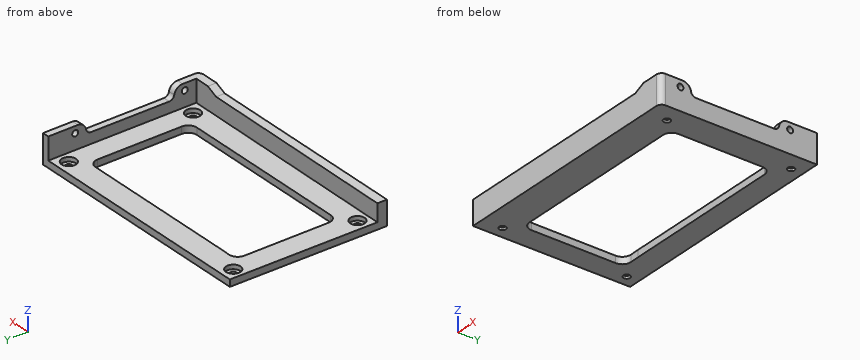
from build123d import *

# Parameters (mm, degrees)
F1_DEPTH  = 17
F3_DEPTH  = 13
F5_R      = 1.75
F6_DEPTH  = 7
F8_DEPTH  = 25
F9_R      = 3
F10_R     = 5
F11_R     = 2
F12_DEPTH = 25
F13_R     = 4.25
F14_DEPTH = 2.5
F16_DEPTH = 25
F17_R     = 5
F18_R     = 3


# Not quite as in the source:
# - ends of sketch curves that miss each other by under 0.0002 mm in the source are joined
# - a feature names something its author has since deleted; it is built from what else it names


with BuildPart() as f1:
    # F0 (on Top) → F1 (new body)
    with BuildSketch(Plane.XY):
        Polygon((67.6393576576, 43.5), (-74.3606423424, 43.5), (-74.7787490059, -48.5), (67.6393576576, -48.5), align=None)
    extrude(amount=F1_DEPTH)

    # F2 (on face) → F3 (cut)
    with BuildSketch(Plane.XY.offset(17)):
        Polygon((63.6393576576, 43.5), (-74.3606423424, 43.5), (-74.7531674957, -42.8710561201), (63.6393576576, -43.5), align=None)
    extrude(amount=-F3_DEPTH, mode=Mode.SUBTRACT)

    # F5 (on face) → F6 (cut)
    with BuildSketch(Plane.YZ.offset(67.6393576576)):
        with Locations((27.6843051805, 13.0568410139)):
            Circle(F5_R)
        with Locations((-36.7146101537, 13.0568410233)):
            Circle(F5_R)
        with BuildLine():
            ThreePointArc((27.6607478596, 17.0567716449), (27.6840839728, 17.0568410078), (27.7074200936, 17.0567742259))
            Line((27.7074200936, 17.0567742259), (47.12958325, 17.057848309))
            Line((47.12958325, 17.057848309), (47.1295543691, 17.7527777587))
            Line((47.1295543691, 17.7527777587), (48.6345604738, 26.1808149253))
            Line((48.6345604738, 26.1808149253), (32.3804893276, 26.9834864621))
            Line((32.3804893276, 26.9834864621), (-57.0169261912, 27.2844880555))
            Line((-57.0169261912, 27.2844880555), (-57.1818195967, 17.0567789567))
            Line((-57.1818195967, 17.0567789567), (-36.7146222837, 17.0568410232))
            Line((-36.7146222837, 17.0568410232), (-30.4415900066, 17.0568410232))
            Line((-30.4415900066, 17.0568410232), (-30.4415900066, 10.3634270296))
            Line((-30.4415900066, 10.3634270296), (21.2007000848, 10.3634270296))
            Line((21.2007000848, 10.3634270296), (21.2007000848, 17.0567742259))
            Line((21.2007000848, 17.0567742259), (27.6607478596, 17.0567716449))
        make_face()
    extrude(amount=-F6_DEPTH, mode=Mode.SUBTRACT)

    # F7 (on face) → F8 (cut)
    with BuildSketch(Plane.XY.offset(4)):
        Polygon((-50.4835, -29.7545), (50.4835, -29.7545), (50.4835, 29.7545), (-50.4835, 29.7545), (-61.1949004233, 29.9527719617), (-61.1949004233, -29.7545), align=None)
    extrude(amount=-F8_DEPTH, mode=Mode.SUBTRACT)

    # F9
    f9_edges = [f1.edges().sort_by_distance(p)[0] for p in [
        (67.639358, -48.5, 8.5),
    ]]
    fillet(f9_edges, radius=F9_R)

    # F10
    f10_edges = [f1.edges().sort_by_distance(p)[0] for p in [
        (50.4835, 29.7545, 2),
        (-61.1949, 29.952772, 2),
        (50.4835, -29.7545, 2),
        (-61.1949, -29.7545, 2),
    ]]
    fillet(f10_edges, radius=F10_R)

    # F11 (on face) → F12 (cut)
    with BuildSketch(Plane.XY.offset(4)):
        with Locations((-67.8764981099, -36.4826410897)):
            Circle(F11_R)
        with Locations((57.0614288288, -36.4826410897)):
            Circle(F11_R)
        with Locations((-67.8764981099, 36.4826410897)):
            Circle(F11_R)
        with Locations((57.0614288288, 36.4826410897)):
            Circle(F11_R)
    extrude(amount=-F12_DEPTH, mode=Mode.SUBTRACT)

    # F13 (on face) → F14 (cut)
    with BuildSketch(Plane.XY.offset(4)):
        with Locations((-67.8764981099, 36.4826410897)):
            Circle(F13_R)
        with Locations((57.0614288288, 36.4826410897)):
            Circle(F13_R)
        with Locations((-67.8764981099, -36.4826410897)):
            Circle(F13_R)
        with Locations((57.0614288288, -36.4826410897)):
            Circle(F13_R)
    extrude(amount=-F14_DEPTH, mode=Mode.SUBTRACT)

    # F15 (on face) → F16 (cut)
    with BuildSketch(Plane.XZ.offset(48.5)):
        Polygon((-78.4085690975, 22.2279634327), (-78.4085690975, 14.2272571102), (48.5201984959, 14.2272571102), (54.7997877002, 17), (47.9935184121, 22.2279634327), align=None)
    extrude(amount=-F16_DEPTH, mode=Mode.SUBTRACT)

    # F17
    f17_edges = [f1.edges().sort_by_distance(p)[0] for p in [
        (65.639358, -30.44159, 17),
        (65.639358, 21.2007, 17),
    ]]
    fillet(f17_edges, radius=F17_R)

    # F18
    f18_edges = [f1.edges().sort_by_distance(p)[0] for p in [
        (65.639358, -30.44159, 10.363427),
        (65.639358, 21.2007, 10.363427),
    ]]
    fillet(f18_edges, radius=F18_R)


solid = f1.part
The listing builds one solid part. Answer for the finished solid, in the listing's coordinates (mm). Coordinates: 2 decimals unless noted, no trailing zeros. Loops run counter-clockwise (first coordinate to the right, second up) from the corner with the lowest first, then second, coordinate; pieces in that order, holes last. Notation, with made-up numbers: (3.5, 78.5) -> (52.5, 78.5) arc R27 cw to (52.5, 113.5) -> close; hole circle Ø4 at (-8.5, 7). An arc over 180 degrees is marked (long way). Write item = value, one per line. Start each with the question number.
1) A cutting plane is placed at A-A (y = 6.5). Give the vertices of the cut face in (x, z), then the cut area to 3 significant figures.
2) Straight lines are drawn through the part: line 1 (Y direction, x = 22, z = 2.5); line 2 (X direction, y = -42, z = 13); line 3 (X direction, y = -28.5, z = 2.5). For each, find the intervals that lie inside material, in ascending order. Write a range as from..to.
3) A cutting plane is placed at C-C (z = 6). Give the vertices of the cut face in (x, y), then the cut area to 3 significant figures.
4) Given pin 1 Ø9.5 at (x, y) = (57.5, -37.5) entering from +Z; pin 2 Ø3 at (x, z) = (37.5, 8.5) entering from +Y; pin 3 Ø1.2 at (x, y) = (66, 0) entering from +Z, each flat-ended and moving along its own axis, determine where each tip first touches the part or whether it passes through.
5) A cutting plane is placed at B-B (x = -2). Give the vertices of the cut face in (y, z), then the cut area to 3 significant figures.
Responses:
q1.outline = (-74.53, 0) -> (-61.19, 0) -> (-61.19, 4) -> (-74.53, 4) -> close; (50.48, 0) -> (67.64, 0) -> (67.64, 10.36) -> (63.64, 10.36) -> (63.64, 4) -> (50.48, 4) -> close
q1.area = 147 mm²
q2.line_1 = -48.5..-29.75, 29.75..43.5
q2.line_2 = 63.64..67.64
q2.line_3 = -74.69..-59.51, 48.8..67.64
q3.outline = (-74.78, -48.5) -> (64.64, -48.5) arc R3 ccw to (67.64, -45.5) -> (67.64, 43.5) -> (63.64, 43.5) -> (63.64, -43.5) -> (-74.75, -42.87) -> close
q3.area = 1,100 mm²
q4.pin_1 = 4
q4.pin_2 = -43.37
q4.pin_3 = 10.36
q5.outline = (-48.5, 0) -> (-29.75, 0) -> (-29.75, 4) -> (-43.2, 4) -> (-43.2, 14.23) -> (-48.5, 14.23) -> close; (29.75, 0) -> (43.5, 0) -> (43.5, 4) -> (29.75, 4) -> close
q5.area = 184 mm²
